Check sheet for the modelled part. Datum: model origin and axes. Units: mm. A direction names the side the tool comes from. Round coordinates to 2 decimals unless told otherwise and drop trailing zeros. Order: outer loops, then holes, each group sorted by start corner. A loop starts at its lowest first (then second) coordinate and runs counter-clockwise, first axis right, second up. Notation, with made-up numbers: M 20,62 L 54,62 A31 cw 54,97 Z; hole C 89.25,19 d2. An arc over 180 degrees is marked long. One line per item, written item: value. Start each with the question number.
(1) Access from +Z, -Z, +X, -X, +Y, -Y to the whole of each face (thin tool, end or side, straight path). Record for faces 5 (the face through (-18.129, -10.263, 14.521)), 6 (the face through (-18.1, -5.57, 14.52)), 7 (the face through (23, 0, 3)).
(2) Thickness scan on L1, parallel to X at y = 0, z = 13.25; L2, parallel to X at y = 0, z = 17.25; L3, parallel to Y at x = 0, z = 18.5. Record the ranges inside material, lowest first.
(3) Depth check by flat-ended pin: pin 1 Ø1 at (x, z) = (-20.5, 6) entering from -Y; pin 2 Ø12 at (x, z) = (17.5, 19.5) entering from +Y; pin 3 Ø11.5 at (x, y) = (-4.5, -19) entering from +Z; pin 4 Ø8 at (x, y) = (-13.5, -3) entering from -Z. Enter the tip coordinate at first touch or a pass-through.
(4) Release check for a two-part mould opening along X. For faces 1 (the face through (-20.293, -11.889, 7.423)), 2 (the face through (22, 0, 19)), 3 (the face through (1.7, -22.1, 0)), 4 (the face through (22.757, 10.351, 8.402)) record: released by +X, released by -X, zero draft, split by the parting line, or undercut.
(5) Cross-section at C-C, the plane z = 5.75. Enter the section's corners in (x, y), and give its area (3 significant figures).
(6) Cross-section at A-A, the plane x = 0. Enter the section's corners in (y, z), and give its area (3 significant figures).
(7) Cross-section at D-D, the plane y = -15.5. Enter the section's corners in (x, z).
Autodesk Fusion 360 part; units mm, degrees
sketch "Sketch1" plane through (0, 0, 0) normal (0, 0, 1) x (1, 0, 0)
  circle A0 centre (0, 0) radius 22
  circle A1 centre (0, 0) radius 25
  dimension "d1" = 44
  dimension "d2" = 50
extrude "Extrude1" add sketch "Sketch1" along normal blind 2 makes body 1
sketch "Sketch2" plane through (0, 0, 2) normal (0, 0, 1) x (-1, 0, 0)
  circle A0 centre (0, 0) radius 22
  circle A1 centre (0, 0) radius 25
  circle A2 centre (0, 0) radius 22
  circle A3 centre (0, 0) radius 25
  line L0 (21.4312, -12.8726) -> (19.1226, -10.8777)
  line L1 (21.4312, 12.8726) -> (19.1226, 10.8777)
  line L2 (-21.4312, -12.8726) -> (-19.1226, -10.8777)
  line L3 (-21.4312, 12.8726) -> (-19.1226, 10.8777)
extrude "Extrude2" add sketch "Sketch2" along normal blind 15 contours A0 A1 A2 A3 L0 L1 | A0 A1 A2 A3 L2 L3 bodies 1
sketch "Sketch3" plane through (0, 0, 17) normal (0, 0, 1) x (-1, 0, 0)
  arc A0 (21.4312, -12.8726) -> (21.4312, 12.8726) centre (0, 0) ccw
  line L0 (21.4312, 12.8726) -> (19.1226, 10.8777)
  arc A1 (19.1226, -10.8777) -> (19.1226, 10.8777) centre (0, 0) ccw
  line L1 (19.1226, -10.8777) -> (21.4312, -12.8726)
  circle A2 centre (0, 0) radius 13.5
  circle A3 centre (0, 0) radius 16.5695
  dimension "d7" = 27
extrude "Extrude3" add sketch "Sketch3" along normal blind 5 separate body contours A3 makes body 2
extrude "Extrude4" add 2 faces at (-23.9039, -1.6648, 17) (23.9039, 1.6648, 17) along direction (0, 0, 1) blind 5 on bodies 1 bodies 1
extrude "Extrude5" add 1 faces at (-15.4344, 1.4939, 17) along direction (0, 0, -1) blind 7 on bodies 2 bodies 2
extrude "Extrude6" cut 2 faces at (-23.9039, -1.6648, 22) (-23.9039, -1.6648, 22) along direction (0, 0, -1) blind 6 on bodies 1 bodies 1
sketch "Sketch4" plane through (0, 0, 16) normal (0, 0, 1) x (-1, 0, 0)
  arc A0 (21.4312, -12.8726) -> (21.4312, 12.8726) centre (0, 0) ccw
  line L0 (21.4312, 12.8726) -> (19.1226, 10.8777)
  arc A1 (19.1226, -10.8777) -> (19.1226, 10.8777) centre (0, 0) ccw
  line L1 (19.1226, -10.8777) -> (21.4312, -12.8726)
  line L2 (21.4312, 12.8726) -> (14, 7)
  line L3 (14, 7) -> (14, -6.4511)
  line L4 (14, -6.4511) -> (21.4312, -12.8726)
extrude "Extrude7" add sketch "Sketch4" against normal blind 3 contours L0 A1 L2 L3 L4 bodies 1 2
mirror "Mirror1" about plane through (0, 0, 0) normal (1, 0, 0) of "Extrude7"
sketch "Sketch5" plane through (0, 0, 0) normal (1, 0, 0) x (0, 1, 0)
  line L0 (-10, 10) -> (10, 10)
  line L1 (10, 10) -> (10, 3)
  line L2 (10, 3) -> (-10, 3)
  line L3 (-10, 3) -> (-10, 10)
extrude "Extrude8" cut sketch "Sketch5" along normal mid plane 54 bodies 1
sketch "Sketch6" plane through (0, 0, 16) normal (0, 0, 1) x (-1, 0, 0)
  arc A0 (21.4312, -12.8726) -> (21.4312, 12.8726) centre (0, 0) ccw
  line L0 (21.4312, 12.8726) -> (14.734, 7.5801)
  arc A1 (14.9067, -7.2346) -> (14.734, 7.5801) centre (0, 0) ccw
  line L1 (14.9067, -7.2346) -> (21.4312, -12.8726)
  circle A2 centre (0, 0) radius 16.5695
  circle A3 centre (0, 0) radius 21.3776
  line L2 (-20.1345, 7.1834) -> (-15.9102, 4.6275)
  line L3 (-20.3781, -6.4601) -> (-16.05, -4.1167)
  line L4 (15.9696, 4.4183) -> (20.2828, 6.7535)
  line L5 (16.1229, -3.8213) -> (20.3951, -6.4063)
extrude "Extrude9" cut sketch "Sketch6" against normal blind 8 contours A2 A3 L2 L3 | A1 A2 A3 L4 L5 bodies 1
Values found:
1. face 5: +Z, -Y
1. face 6: +Z, -Z
1. face 7: +X, -X
2. L1: -25 to -21.38, -16.57 to -13.5, 13.5 to 16.57, 21.38 to 25
2. L2: -16.57 to -13.5, 13.5 to 16.57, 22 to 25
2. L3: -16.57 to -13.5, 13.5 to 16.57
3. pin 1: y = -12.5
3. pin 2: y = 12.87
3. pin 3: z = 22
3. pin 4: z = 10
4. face 1: undercut
4. face 2: undercut
4. face 3: zero draft
4. face 4: split by the parting line
5. outline: M -22.91,-10 A25 ccw -21.43,-12.87 L -19.12,-10.88 A22 cw -19.6,-10 Z; M -22.91,10 L -19.6,10 A22 cw -19.12,10.88 L -21.43,12.87 A25 ccw Z; M 19.12,-10.88 L 21.43,-12.87 A25 ccw 22.91,-10 L 19.6,-10 A22 cw Z; M 19.12,10.88 A22 cw 19.6,10 L 22.91,10 A25 ccw 21.43,12.87 Z
5. area: 25.4 mm^2
6. outline: M -25,0 L -22,0 L -22,2 L -25,2 Z; M -16.57,10 L -13.5,10 L -13.5,22 L -16.57,22 Z; M 13.5,10 L 16.57,10 L 16.57,22 L 13.5,22 Z; M 22,0 L 25,0 L 25,2 L 22,2 Z
6. area: 85.7 mm^2
7. outline: M -19.62,0 L -15.61,0 L -15.61,2 L -19.62,2 Z; M -5.86,10 L 5.86,10 L 5.86,22 L -5.86,22 Z; M 15.61,0 L 19.62,0 L 19.62,2 L 15.61,2 Z
